Work out the finished part from the listing and answer in its coordinate system (mm). Face numbers are marked on the shaded views. A direction names the side the tool comes from. Coordinates: 2 decimals unless noted, no trailing zeros. Order: outer loops, then holes, each group sorted by start corner. A loop starts at its lowest first (then second) coordinate and runs counter-clockwise, first axis right, second up. Notation, with made-up numbers: (5, 48) -> (63, 48) arc R12 cw to (63, 52) -> close; hole circle Ø6 at (24.5, -34.5). An arc over 180 degrees is marked (long way). Use one line per item in the form item = value.
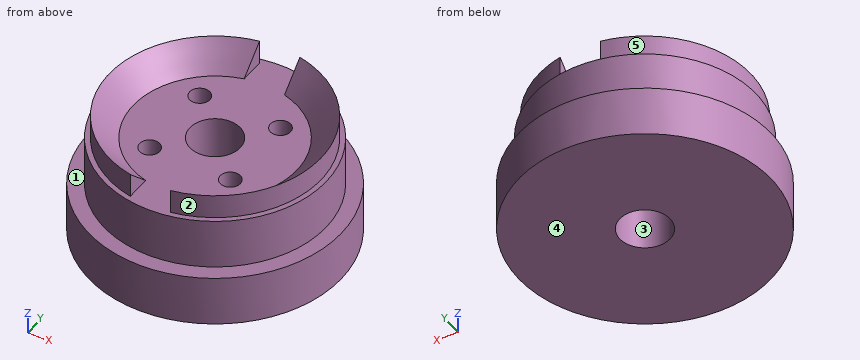
from build123d import *

# Parameters (mm, degrees)
F0_R        = 12.5
F0_R_2      = 11
F1_DEPTH    = 5
F0_R_3      = 1
F2_DEPTH    = 10
F3_DEPTH    = 15
F4_T4_ANGLE = 333.3635987438
F4_T9_ANGLE = 333.3635987438
F5_D        = 5
F5_DEPTH    = 12
F5_TIP      = 1.5021515476
F6_DEPTH    = 8


# Not quite as in the source:
# - a fillet or chamfer that OpenCascade refuses, or shapes differently, is made with other operations: its cross-section is extruded or revolved along the edge and cut away or added


with BuildPart() as f1:
    # F0 (on Top) → F1 (new body)
    with BuildSketch(Plane.XY):
        Circle(F0_R)
        Circle(F0_R_2, mode=Mode.SUBTRACT)
    extrude(amount=F1_DEPTH)

    # F0 (on Top) → F2 (join)
    with BuildSketch(Plane.XY):
        Circle(F0_R_2)
        with Locations((-4, -4)):
            Circle(F0_R_3, mode=Mode.SUBTRACT)
        with Locations((4, -4)):
            Circle(F0_R_3, mode=Mode.SUBTRACT)
        with BuildLine():
            ThreePointArc((-2, -10.307764064), (-10.5, 0), (-2, 10.307764064))
            Line((-2, 10.307764064), (-2, 7.8581159461))
            ThreePointArc((-2, 7.8581159461), (-8.1086365206, 0), (-2, -7.8581159461))
            Line((-2, -7.8581159461), (-2, -10.307764064))
        make_face(mode=Mode.SUBTRACT)
        with Locations((-4, 4)):
            Circle(F0_R_3, mode=Mode.SUBTRACT)
        with Locations((4, 4)):
            Circle(F0_R_3, mode=Mode.SUBTRACT)
        with BuildLine():
            ThreePointArc((2, 10.307764064), (10.5, 0), (2, -10.307764064))
            Line((2, -10.307764064), (2, -7.8581159461))
            ThreePointArc((2, -7.8581159461), (8.1086365206, 0), (2, 7.8581159461))
            Line((2, 7.8581159461), (2, 10.307764064))
        make_face(mode=Mode.SUBTRACT)
    extrude(amount=F2_DEPTH)

    # F0 (on Top) → F3 (join)
    with BuildSketch(Plane.XY):
        with BuildLine():
            Line((-2, 7.8581159461), (-2, 10.307764064))
            ThreePointArc((-2, 10.307764064), (-10.5, 0), (-2, -10.307764064))
            Line((-2, -10.307764064), (-2, -7.8581159461))
            ThreePointArc((-2, -7.8581159461), (-8.1086365206, 0), (-2, 7.8581159461))
        make_face()
        with BuildLine():
            Line((2, -7.8581159461), (2, -10.307764064))
            ThreePointArc((2, -10.307764064), (10.5, 0), (2, 10.307764064))
            Line((2, 10.307764064), (2, 7.8581159461))
            ThreePointArc((2, 7.8581159461), (8.1086365206, 0), (2, -7.8581159461))
        make_face()
    extrude(amount=F3_DEPTH)

    # F4: chamfer of 5 on 2 edges, made by hand


with BuildPart() as f4_tool2:
    # F4_s3 → F4_t4 (revolve)
    with BuildSketch(Plane(origin=(0, 0, 0), x_dir=(0, 0, 1), z_dir=(0.2303588664, 0.9731057459, 0))):
        Polygon((10, 8.1086365206), (15, 13.1086365206), (15, 8.1086365206), align=None)
    revolve(axis=Axis((0, 0, 15), (0, 0, -1)), revolution_arc=F4_T4_ANGLE)

    split(bisect_by=Plane.XY.offset(10), keep=Keep.TOP)


with BuildPart() as f1_1:
    add(f1.part)

    # F4_t1: cut F4_tool2
    add(f4_tool2.part, mode=Mode.SUBTRACT)


with BuildPart() as f4_tool7:
    # F4_s8 → F4_t9 (revolve)
    with BuildSketch(Plane(origin=(0, 0, 0), x_dir=(0, 0, 1), z_dir=(-0.2303588664, -0.9731057459, 0))):
        Polygon((10, 8.1086365206), (15, 13.1086365206), (15, 8.1086365206), align=None)
    revolve(axis=Axis((0, 0, 15), (0, 0, -1)), revolution_arc=F4_T9_ANGLE)

    split(bisect_by=Plane.XY.offset(10), keep=Keep.TOP)


with BuildPart() as f1_2:
    add(f1_1.part)

    # F4_t6: cut F4_tool7
    add(f4_tool7.part, mode=Mode.SUBTRACT)

    # F5
    with Locations(Plane(origin=(0, 0, 0), x_dir=(1, 0, 0), z_dir=(0, 0, -1))):
        with Locations((0, 0)):
            Hole(F5_D / 2, depth=F5_DEPTH)
            with Locations((0, 0, -(F5_DEPTH + F5_TIP / 2))):  # 118° drill point
                Cone(0, F5_D / 2, F5_TIP, mode=Mode.SUBTRACT)

    # F0 (on Top) → F6 (join)
    with BuildSketch(Plane.XY):
        with Locations((-4, 4)):
            Circle(F0_R_3)
        with Locations((4, 4)):
            Circle(F0_R_3)
        with Locations((-4, -4)):
            Circle(F0_R_3)
        with Locations((4, -4)):
            Circle(F0_R_3)
    extrude(amount=F6_DEPTH)


solid = f1_2.part
(1) Straight lines are drawn through the part: line 1 along Y through (x, z) = (4, 9.25); line 2 along Y through (x, z) = (0, 3.25); line 3 along Z through (x, y) = (10, -5.25). For each, find the intervals that lie inside material, in ascending order.
Data:
line_1 = -10.25 to -5, -3 to 3, 5 to 10.25
line_2 = -12.5 to -2.5, 2.5 to 12.5
line_3 = 0 to 5
(2) Each of these flat-tipped pins is pushed along its axis until it touches: P1, Ø5, axis at y = -9, z = 10, coming from the +X side; P2, Ø6, axis at y = 4, z = 9, coming from the -X side; P3, Ø1.5, axis at x = -6.5, z = 10, coming from the -Y side. Where does it stop, or does it pass through?
Data:
P1 = 8.87
P2 = -10.95
P3 = -9.38
(3) Section B-B on y = 0 is taken. Write down the section's boundary in (x, z), plus the area to 3 significant figures.
Data:
outline = (-12.5, 0) -> (-2.5, 0) -> (-2.5, 10) -> (-8.11, 10) -> (-10.5, 12.39) -> (-10.5, 10) -> (-11, 10) -> (-11, 5) -> (-12.5, 5) -> close; (2.5, 0) -> (12.5, 0) -> (12.5, 5) -> (11, 5) -> (11, 10) -> (10.5, 10) -> (10.5, 12.39) -> (8.11, 10) -> (2.5, 10) -> close
area = 191 mm²
(4) Which of the six approach directions +Z, -Z, +X, -X, +Y, -Y give full straight-line access (tool end or side, diameter ignored) to the marked faces 1, 2, 3, 4 and 5?
Data:
face_1 = +Z
face_2 = +Z, +X
face_3 = +Z, -Z
face_4 = -Z, +X, -X, +Y, -Y
face_5 = +Z, -X
(5) Section C-C on z = 10.5 is taken. Write down the section's boundary in (x, y), plus the area to 3 significant figures.
Data:
outline = (-2, -10.31) -> (-2, -8.37) arc R8.61 cw to (-2, 8.37) -> (-2, 10.31) arc R10.5 ccw to start; (2, -10.31) arc R10.5 ccw to (2, 10.31) -> (2, 8.37) arc R8.61 cw to (2, -8.37) -> close
area = 98.3 mm²
(6) Section D-D on z = 2.25 is taken. Write down the section's boundary in (x, y), plus the area to 3 significant figures.
Data:
outline = circle Ø25 at (0, 0); hole circle Ø5 at (0, 0)
area = 471 mm²
(7) Section A-A on x = 0 is taken. Write down the section's boundary in (y, z).
Data:
outline = (-12.5, 0) -> (-2.5, 0) -> (-2.5, 10) -> (-11, 10) -> (-11, 5) -> (-12.5, 5) -> close; (2.5, 0) -> (12.5, 0) -> (12.5, 5) -> (11, 5) -> (11, 10) -> (2.5, 10) -> close
